Geometry: final body of the model. Coordinates: model frame, mm. Face numbers are marked on the shaded views. A direction names the side the tool comes from. Coordinates: 2 decimals unless noted, no trailing zeros. Write each loop counter-clockwise with the first axis right and the second up, starting at its lowest first coordinate (ties: lowest second). Pieces come first, ordered by that corner, then holes. Notation, with made-up numbers: (37, 30.5) - (66, 30.5) arc R31 ccw to (66, 59.5) - close; hole circle Ø9 at (-4, 24.5). An arc over 180 degrees is marked (long way). Answer as a JSON object with one key per item and string values. Group by question number.
Item 1: Line query: line 1 along Z through (x, y) = (7.25, 0.25); line 2 along Z through (x, y) = (4, -8); line 3 along Y through (x, z) = (0, -7.5). Output: solid intervals per line, ascending. Write a range as from..to.
Item 2: Section A-A on x = 0. Return loops of the section in (y, z), and give its area (3 significant figures).
Item 3: First-contact query: pin 1 Ø8 at (y, z) = (6, -7.5) entering from -X; pin 2 Ø0.6 at (x, z) = (0, -1.5) entering from +Y; pin 3 Ø1 at (y, z) = (-7.5, -4.5) entering from -X. Flat tips, straight axial feed; report the tip coordinate or a pass-through.
Item 4: Section B-B on z = -6.5. Return loops of the section in (x, y), and give its area (3 significant figures).
Item 5: Set-up query: the marked faces 1 and 2. Return all of +Z, -Z, +X, -X, +Y, -Y with unobstructed straight access to the full face (end or side cutting, diameter ignored); none if empty.
Item 6: Mould query, pull axis Y, two halves, no side actions, for the marked faces 3, 4 and 5. Classes: pulls with the +Y half, pulls with the -Y half, needs draft (parallel to the pull), parting line crosses it, or undercut.
```python
from build123d import *

# Parameters (mm, degrees)
BOSS_EXTRUDE1_DEPTH = 5
SKETCH2_R           = 10
BOSS_EXTRUDE2_DEPTH = 1
SKETCH4_R           = 6
BOSS_EXTRUDE3_DEPTH = 5
CUT_EXTRUDE1_REACH  = 17
SKETCH5_R           = 2.75
SKETCH7_R           = 8.1
CUT_EXTRUDE2_DEPTH  = 2.6


with BuildPart() as part:
    # Sketch1 → Boss-Extrude1 (new body, symmetric)
    with BuildSketch(Plane.XY):
        with BuildLine():
            Line((-0.4, 9.191300234), (-0.660980834, 8.474261286))
            ThreePointArc((-0.660980834, 8.474261286), (-1.065332485, 8.432974961), (-1.467248177, 8.372406033))
            Line((-1.467248177, 8.372406033), (-1.898350154, 9.002014591))
            Line((-1.898350154, 9.002014591), (-2.673216683, 8.803062681))
            Line((-2.673216683, 8.803062681), (-2.747677989, 8.043647535))
            ThreePointArc((-2.747677989, 8.043647535), (-3.129058698, 7.90310013), (-3.503284589, 7.744481718))
            Line((-3.503284589, 7.744481718), (-4.077419986, 8.247099263))
            Line((-4.077419986, 8.247099263), (-4.77846533, 7.861696324))
            Line((-4.77846533, 7.861696324), (-4.66172843, 7.107621828))
            ThreePointArc((-4.66172843, 7.107621828), (-4.996174644, 6.876644452), (-5.319196746, 6.629943135))
            Line((-5.319196746, 6.629943135), (-6.000290524, 6.973988359))
            Line((-6.000290524, 6.973988359), (-6.583465426, 6.426350674))
            Line((-6.583465426, 6.426350674), (-6.282865329, 5.724998101))
            ThreePointArc((-6.282865329, 5.724998101), (-6.549362564, 5.418103913), (-6.80088421, 5.098820841))
            Line((-6.80088421, 5.098820841), (-7.546140742, 5.262676117))
            Line((-7.546140742, 5.262676117), (-7.974802178, 4.587213776))
            Line((-7.974802178, 4.587213776), (-7.509226693, 3.982651688))
            ThreePointArc((-7.509226693, 3.982651688), (-7.691029946, 3.619123978), (-7.855247106, 3.247320882))
            Line((-7.855247106, 3.247320882), (-8.617839183, 3.220690579))
            Line((-8.617839183, 3.220690579), (-8.865052779, 2.459845366))
            Line((-8.865052779, 2.459845366), (-8.263755727, 1.990060623))
            ThreePointArc((-8.263755727, 1.990060623), (-8.349441631, 1.592741174), (-8.416035937, 1.191779808))
            Line((-8.416035937, 1.191779808), (-9.148047095, 0.976337208))
            Line((-9.148047095, 0.976337208), (-9.198279511, 0.177915826))
            Line((-9.198279511, 0.177915826), (-8.499042597, -0.127573271))
            ThreePointArc((-8.499042597, -0.127573271), (-8.483227192, -0.533719416), (-8.448014278, -0.938645173))
            Line((-8.448014278, -0.938645173), (-9.103449564, -1.32936302))
            Line((-9.103449564, -1.32936302), (-8.953544512, -2.115192821))
            Line((-8.953544512, -2.115192821), (-8.200303363, -2.237191266))
            ThreePointArc((-8.200303363, -2.237191266), (-8.083980389, -2.626644452), (-7.949172812, -3.010091627))
            Line((-7.949172812, -3.010091627), (-8.486848816, -3.551534481))
            Line((-8.486848816, -3.551534481), (-8.146225383, -4.275396123))
            Line((-8.146225383, -4.275396123), (-7.38630891, -4.206238307))
            ThreePointArc((-7.38630891, -4.206238307), (-7.176787367, -4.554527757), (-6.950855584, -4.892402953))
            Line((-6.950855584, -4.892402953), (-7.336988145, -5.550549969))
            Line((-7.336988145, -5.550549969), (-6.827048953, -6.166960564))
            Line((-6.827048953, -6.166960564), (-6.108205503, -5.910991925))
            ThreePointArc((-6.108205503, -5.910991925), (-5.8186504, -6.196233333), (-5.515790536, -6.467306608))
            Line((-5.515790536, -6.467306608), (-5.726117525, -7.200803989))
            Line((-5.726117525, -7.200803989), (-5.078903929, -7.671032191))
            Line((-5.078903929, -7.671032191), (-4.44630108, -7.244336181))
            ThreePointArc((-4.44630108, -7.244336181), (-4.09490623, -7.44860678), (-3.734148082, -7.635845605))
            Line((-3.734148082, -7.635845605), (-3.755453882, -8.398605012))
            Line((-3.755453882, -8.398605012), (-3.011632693, -8.693104654))
            Line((-3.011632693, -8.693104654), (-2.505019208, -8.122492153))
            ThreePointArc((-2.505019208, -8.122492153), (-2.113864041, -8.23295687), (-1.717875372, -8.324596339))
            Line((-1.717875372, -8.324596339), (-1.54882126, -9.068690793))
            Line((-1.54882126, -9.068690793), (-0.755129499, -9.16895738))
            Line((-0.755129499, -9.16895738), (-0.406337766, -8.49028207))
            ThreePointArc((-0.406337766, -8.49028207), (0, -8.5), (0.406337766, -8.49028207))
            Line((0.406337766, -8.49028207), (0.755129499, -9.16895738))
            Line((0.755129499, -9.16895738), (1.54882126, -9.068690793))
            Line((1.54882126, -9.068690793), (1.717875372, -8.324596339))
            ThreePointArc((1.717875372, -8.324596339), (2.113864041, -8.23295687), (2.505019208, -8.122492153))
            Line((2.505019208, -8.122492153), (3.011632693, -8.693104654))
            Line((3.011632693, -8.693104654), (3.755453882, -8.398605012))
            Line((3.755453882, -8.398605012), (3.734148082, -7.635845605))
            ThreePointArc((3.734148082, -7.635845605), (4.09490623, -7.44860678), (4.44630108, -7.244336181))
            Line((4.44630108, -7.244336181), (5.078903929, -7.671032191))
            Line((5.078903929, -7.671032191), (5.726117525, -7.200803989))
            Line((5.726117525, -7.200803989), (5.515790536, -6.467306608))
            ThreePointArc((5.515790536, -6.467306608), (5.8186504, -6.196233333), (6.108205503, -5.910991925))
            Line((6.108205503, -5.910991925), (6.827048953, -6.166960564))
            Line((6.827048953, -6.166960564), (7.336988145, -5.550549969))
            Line((7.336988145, -5.550549969), (6.950855584, -4.892402953))
            ThreePointArc((6.950855584, -4.892402953), (7.176787367, -4.554527757), (7.38630891, -4.206238307))
            Line((7.38630891, -4.206238307), (8.146225383, -4.275396123))
            Line((8.146225383, -4.275396123), (8.486848816, -3.551534481))
            Line((8.486848816, -3.551534481), (7.949172812, -3.010091627))
            ThreePointArc((7.949172812, -3.010091627), (8.083980389, -2.626644452), (8.200303363, -2.237191266))
            Line((8.200303363, -2.237191266), (8.953544512, -2.115192821))
            Line((8.953544512, -2.115192821), (9.103449564, -1.32936302))
            Line((9.103449564, -1.32936302), (8.448014278, -0.938645173))
            ThreePointArc((8.448014278, -0.938645173), (8.483227192, -0.533719416), (8.499042597, -0.127573271))
            Line((8.499042597, -0.127573271), (9.198279511, 0.177915826))
            Line((9.198279511, 0.177915826), (9.148047095, 0.976337208))
            Line((9.148047095, 0.976337208), (8.416035937, 1.191779808))
            ThreePointArc((8.416035937, 1.191779808), (8.349441631, 1.592741174), (8.263755727, 1.990060623))
            Line((8.263755727, 1.990060623), (8.865052779, 2.459845366))
            Line((8.865052779, 2.459845366), (8.617839183, 3.220690579))
            Line((8.617839183, 3.220690579), (7.855247106, 3.247320882))
            ThreePointArc((7.855247106, 3.247320882), (7.691029946, 3.619123978), (7.509226693, 3.982651688))
            Line((7.509226693, 3.982651688), (7.974802178, 4.587213776))
            Line((7.974802178, 4.587213776), (7.546140742, 5.262676117))
            Line((7.546140742, 5.262676117), (6.80088421, 5.098820841))
            ThreePointArc((6.80088421, 5.098820841), (6.549362564, 5.418103913), (6.282865329, 5.724998101))
            Line((6.282865329, 5.724998101), (6.583465426, 6.426350674))
            Line((6.583465426, 6.426350674), (6.000290524, 6.973988359))
            Line((6.000290524, 6.973988359), (5.319196746, 6.629943135))
            ThreePointArc((5.319196746, 6.629943135), (4.996174644, 6.876644452), (4.66172843, 7.107621828))
            Line((4.66172843, 7.107621828), (4.77846533, 7.861696324))
            Line((4.77846533, 7.861696324), (4.077419986, 8.247099263))
            Line((4.077419986, 8.247099263), (3.503284589, 7.744481718))
            ThreePointArc((3.503284589, 7.744481718), (3.129058698, 7.90310013), (2.747677989, 8.043647535))
            Line((2.747677989, 8.043647535), (2.673216683, 8.803062681))
            Line((2.673216683, 8.803062681), (1.898350154, 9.002014591))
            Line((1.898350154, 9.002014591), (1.467248177, 8.372406033))
            ThreePointArc((1.467248177, 8.372406033), (1.065332485, 8.432974961), (0.660980834, 8.474261286))
            Line((0.660980834, 8.474261286), (0.4, 9.191300234))
            Line((0.4, 9.191300234), (-0.4, 9.191300234))
        make_face()
    extrude(amount=BOSS_EXTRUDE1_DEPTH, both=True)

    # Sketch2 → Boss-Extrude2 (add)
    with BuildSketch(Plane.XY.offset(5)):
        Circle(SKETCH2_R)
    boss_extrude2 = extrude(amount=-BOSS_EXTRUDE2_DEPTH)

    # Mirror1: Boss-Extrude2 across plane
    add(boss_extrude2.mirror(Plane.XY))

    # Sketch4 → Boss-Extrude3 (add)
    with BuildSketch(Plane(origin=(0, 0, -5), x_dir=(-1, 0, 0), z_dir=(0, 0, -1))):
        Circle(SKETCH4_R)
    extrude(amount=BOSS_EXTRUDE3_DEPTH)

    # Sketch5 → Cut-Extrude1 (cut, up to next)
    with BuildSketch(Plane.XY.offset(5), mode=Mode.PRIVATE) as cut_extrude1_sk1:
        Circle(SKETCH5_R)
    cut_extrude1_tool1 = extrude(cut_extrude1_sk1.sketch, amount=-CUT_EXTRUDE1_REACH, mode=Mode.PRIVATE) & part.part
    add(cut_extrude1_tool1.solids().sort_by_distance((0, 0, 5))[0], mode=Mode.SUBTRACT)

    # Sketch7 → Cut-Extrude2 (cut, symmetric)
    with BuildSketch(Plane.XY):
        Circle(SKETCH7_R)
    extrude(amount=CUT_EXTRUDE2_DEPTH, both=True, mode=Mode.SUBTRACT)


solid = part.part
```
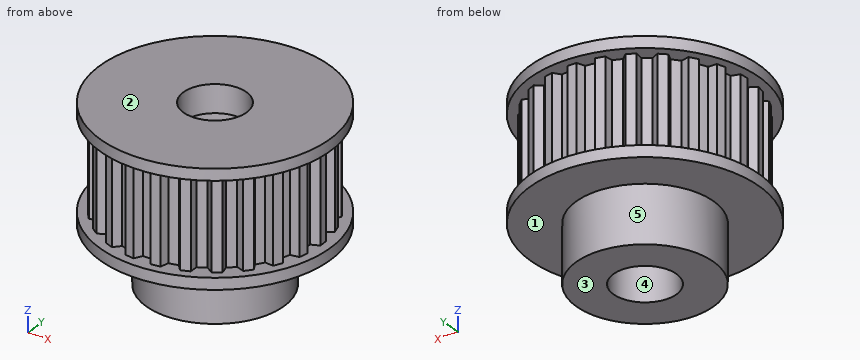
Checks:
{
 "1": {"line 1": "-5..-2.6, 2.6..5", "line 2": "-5..-4, 4..5", "line 3": "-6..-2.75, 2.75..6"},
 "2": {"outline": "(-10, -5) - (-6, -5) - (-6, -10) - (-2.75, -10) - (-2.75, -2.6) - (-8.1, -2.6) - (-8.1, 2.6) - (-2.75, 2.6) - (-2.75, 5) - (-10, 5) - (-10, 4) - (-8.5, 4) - (-8.5, -4) - (-10, -4) - close; (2.75, -10) - (6, -10) - (6, -5) - (10, -5) - (10, -4) - (9.19, -4) - (9.19, 4) - (10, 4) - (10, 5) - (2.75, 5) - (2.75, 2.6) - (8.1, 2.6) - (8.1, -2.6) - (2.75, -2.6) - close", "area": "103 mm^2"},
 "3": {"pin 1": "x = -9.58", "pin 2": "y = 9.19", "pin 3": "x = -7.14"},
 "4": {"outline": "circle Ø12 at (0, 0); hole circle Ø5.5 at (0, 0)", "area": "89.3 mm^2"},
 "5": {"face 1": "-Z", "face 2": "+Z, +X, -X, +Y, -Y"},
 "6": {"face 3": "needs draft", "face 4": "undercut", "face 5": "parting line crosses it"}
}
